```python
from build123d import *

# Parameters (mm, degrees)
SKETCH1_W           = 166
SKETCH1_H           = 88
BOSS_EXTRUDE1_DEPTH = 32
SKETCH2_R           = 44
SKETCH2_R_2         = 25
BOSS_EXTRUDE2_DEPTH = 56
SKETCH3_R           = 16
BOSS_EXTRUDE3_DEPTH = 28


with BuildPart() as part:
    # Sketch1 → Boss-Extrude1 (new body)
    with BuildSketch(Plane(origin=(0, 0, 0), x_dir=(1, 0, 0), z_dir=(0, 1, 0))):
        Rectangle(SKETCH1_W, SKETCH1_H)
    extrude(amount=BOSS_EXTRUDE1_DEPTH)

    # Sketch2 → Boss-Extrude2 (add)
    with BuildSketch(Plane(origin=(0, 32, 0), x_dir=(1, 0, 0), z_dir=(0, 1, 0))):
        with Locations(Location((0, 0, 0), (0, 0, 270))):
            Circle(SKETCH2_R)
        with Locations(Location((0, 0, 0), (0, 0, 270))):
            Circle(SKETCH2_R_2, mode=Mode.SUBTRACT)
    extrude(amount=BOSS_EXTRUDE2_DEPTH)

    # Sketch3 → Boss-Extrude3 (add)
    with BuildSketch(Plane(origin=(83, 0, 0), x_dir=(0, 0, -1), z_dir=(1, 0, 0))):
        with BuildLine():
            Line((-37.732085488, -52.504411697), (-44, 0))
            Line((-44, 0), (44, 0))
            Line((44, 0), (37.732085488, -52.504411697))
            ThreePointArc((37.732085488, -52.504411697), (0, -86), (-37.732085488, -52.504411697))
        make_face()
        with Locations((0, -48)):
            Circle(SKETCH3_R, mode=Mode.SUBTRACT)
    boss_extrude3 = extrude(amount=-BOSS_EXTRUDE3_DEPTH)

    # Mirror1: Boss-Extrude3 across plane
    add(boss_extrude3.mirror(Plane(origin=(0, 0, 0), x_dir=(0, 0, 1), z_dir=(1, 0, 0))))


solid = part.part
```
Design review of the part built by this model. Coordinates are the model's own, in mm. A direction names the side the tool comes from. Round coordinates to 2 decimals unless told otherwise and drop trailing zeros. Write each loop counter-clockwise with the first axis right and the second up, starting at its lowest first coordinate (ties: lowest second). Pieces come first, ordered by that corner, then holes.
Item 1: We need section C-C on x = -63. Write out the cut boundary in (y, z).
Item 2: The part is to be moulded in two halves that separate along X. For faces 1 (the flat face through (-83, -13, -1)), 2 (the cylindrical face through (7.509, 59.608, 23.846)), 3 (the flat face through (-69.2, -25.88, -40.91)), say which applies: +X half, -X half, draft (parallel to the pull), parting line (faces both ways), or undercut.
Item 3: We need section D-D on y = 41.5. Write out the cut boundary in (x, z).
Item 4: We need section B-B on y = -9.5. Write out the cut boundary in (x, z), and give its area (3 significant figures).
Item 5: We need section A-A on z = 0. Write out the cut boundary in (x, y).
Item 6: Clearance check with flat-ended pins moving along their axes: pin 1 Ø1 at (x, z) = (58.5, -17) entering from +Y; pin 2 Ø10 at (x, z) = (29, 21) entering from -Y; pin 3 Ø8 at (x, y) = (59.5, -39.5) entering from +Z; pin 4 Ø19 at (y, z) = (-48, 0) entering from -X. State where each tip first meets the part, or that it passes through.
Item 7: For probe 1 along X at (y, z) = (-72, 13); probe 2 along Y at (x, z) = (-69, 0); probe 3 along X at (y, z) = (68.5, 0), list the stretches that pass through material, from the lowest coordinate up.
Item 8: For faces 4 (the flat face through (0, 32, 0)), 5 (the flat face through (-69.196, -26.62, 40.822)), 6 (the flat face through (-1, 0, -1)), list the 3-axis set-ups (+Z, -Z, +X, -X, +Y, -Y) from which the entire face can be reached by the end or side of a thin tool; tool diameter is ignored.
Returned:
1. outline: (-52.5, -37.73) - (0, -44) - (32, -44) - (32, 44) - (0, 44) - (-52.5, 37.73) arc R38 ccw to start; hole circle Ø32 at (-48, 0)
2. face 1: -X half
2. face 2: undercut
2. face 3: draft
3. outline: circle Ø88 at (0, 0); hole circle Ø50 at (0, 0)
4. outline: (-83, -42.87) - (-55, -42.87) - (-55, 42.87) - (-83, 42.87) - close; (55, -42.87) - (83, -42.87) - (83, 42.87) - (55, 42.87) - close
4. area: 4,800 mm2
5. outline: (-83, -86) - (-55, -86) - (-55, -64) - (-83, -64) - close; (-83, -32) - (-55, -32) - (-55, 0) - (55, 0) - (55, -32) - (83, -32) - (83, 32) - (44, 32) - (44, 88) - (25, 88) - (25, 32) - (-25, 32) - (-25, 88) - (-44, 88) - (-44, 32) - (-83, 32) - close; (55, -86) - (83, -86) - (83, -64) - (55, -64) - close
6. pin 1: stops at y = 32
6. pin 2: stops at y = 0
6. pin 3: stops at z = 39.76
6. pin 4: passes through
7. probe 1: x = -83 to -55, 55 to 83
7. probe 2: y = -86 to -64, -32 to 32
7. probe 3: x = -44 to -25, 25 to 44
8. face 4: +Y
8. face 5: +Z, +X, -X, -Y
8. face 6: +Z, -Z, -Y
